from build123d import *

# Parameters (mm, degrees)
BOSS_EXTRUDE1_DEPTH = 19.05
SKETCH3_R           = 24.5745
CUT_EXTRUDE1_DEPTH  = 175.004260005
SKETCH5_R           = 51.3715
SKETCH5_R_2         = 46.5455
CUT_EXTRUDE2_DEPTH  = 2.794
SKETCH19_R          = 1.7272
CUT_EXTRUDE4_DEPTH  = 175.004260005
CIRPATTERN2_COUNT   = 8
SKETCH37_R          = 119.0625
SKETCH37_R_2        = 115.2525
CUT_EXTRUDE7_DEPTH  = 2.667
CIRPATTERN4_COUNT   = 8


with BuildPart() as part:
    # Sketch1 → Boss-Extrude1 (new body)
    with BuildSketch(Plane(origin=(0, 0, 0), x_dir=(1, 0, 0), z_dir=(0, 1, 0))):
        with BuildLine():
            ThreePointArc((-31.932272077, 122.3), (-48.371185851, 116.778372909), (-63.899633215, 109.058685463))
            Line((-63.899633215, 109.058685463), (-109.058685463, 63.899633215))
            ThreePointArc((-109.058685463, 63.899633215), (-116.778372909, 48.371185851), (-122.3, 31.932272077))
            Line((-122.3, 31.932272077), (-122.3, -31.932272077))
            ThreePointArc((-122.3, -31.932272077), (-116.778372909, -48.371185851), (-109.058685463, -63.899633215))
            Line((-109.058685463, -63.899633215), (-63.899633215, -109.058685463))
            ThreePointArc((-63.899633215, -109.058685463), (-48.371185851, -116.778372909), (-31.932272077, -122.3))
            Line((-31.932272077, -122.3), (31.932272077, -122.3))
            ThreePointArc((31.932272077, -122.3), (48.371185851, -116.778372909), (63.899633215, -109.058685463))
            Line((63.899633215, -109.058685463), (109.058685463, -63.899633215))
            ThreePointArc((109.058685463, -63.899633215), (116.778372909, -48.371185851), (122.3, -31.932272077))
            Line((122.3, -31.932272077), (122.3, 31.932272077))
            ThreePointArc((122.3, 31.932272077), (116.778372909, 48.371185851), (109.058685463, 63.899633215))
            Line((109.058685463, 63.899633215), (63.899633215, 109.058685463))
            ThreePointArc((63.899633215, 109.058685463), (48.371185851, 116.778372909), (31.932272077, 122.3))
            Line((31.932272077, 122.3), (-31.932272077, 122.3))
        make_face()
    extrude(amount=BOSS_EXTRUDE1_DEPTH)

    # Sketch3 → Cut-Extrude1 (cut, through all)
    with BuildSketch(Plane(origin=(0, 19.05, 0), x_dir=(1, 0, 0), z_dir=(0, 1, 0))):
        with Locations(Location((0, 0, 0), (0, 0, 270))):
            Circle(SKETCH3_R)
    extrude(amount=-CUT_EXTRUDE1_DEPTH, mode=Mode.SUBTRACT)

    # Sketch5 → Cut-Extrude2 (cut)
    with BuildSketch(Plane(origin=(0, 19.05, 0), x_dir=(1, 0, 0), z_dir=(0, 1, 0))):
        with Locations(Location((0, 0, 0), (0, 0, 270))):
            Circle(SKETCH5_R)
        with Locations(Location((0, 0, 0), (0, 0, 270))):
            Circle(SKETCH5_R_2, mode=Mode.SUBTRACT)
    extrude(amount=-CUT_EXTRUDE2_DEPTH, mode=Mode.SUBTRACT)

    # Sketch19 → Cut-Extrude4 (cut, through all)
    with BuildSketch(Plane(origin=(0, 19.05, 0), x_dir=(1, 0, 0), z_dir=(0, 1, 0))):
        with Locations(Location((-47.055461432, 113.601933173, 0), (0, 0, 270))):
            Circle(SKETCH19_R)
    cut_extrude4 = extrude(amount=-CUT_EXTRUDE4_DEPTH, mode=Mode.SUBTRACT)

    # CirPattern2: Cut-Extrude4 ×8 about axis
    cirpattern2_axis = Axis((0, 0, 0), (0, 1, 0))
    for i in range(1, CIRPATTERN2_COUNT):
        add(cut_extrude4.rotate(cirpattern2_axis, i * 360 / CIRPATTERN2_COUNT), mode=Mode.SUBTRACT)

    # Sketch23 → 5/16-18 Tapped Hole2 (revolve, cut)
    with BuildSketch(Plane(origin=(-71.374, 19.05, 0), x_dir=(0, 0, 1), z_dir=(1, 0, 0))):
        Polygon((0, 0), (0, 14.661148974), (3.2639, 12.7), (3.2639, 0), align=None)
    f_5_16_18_tapped_hole2 = revolve(axis=Axis((-71.374, 25.4, 0), (0, -1, 0)), mode=Mode.SUBTRACT)

    # Sketch37 → Cut-Extrude7 (cut)
    with BuildSketch(Plane.XZ):
        with Locations(Location((0, 0, 0), (0, 0, 270))):
            Circle(SKETCH37_R)
        with Locations(Location((0, 0, 0), (0, 0, 270))):
            Circle(SKETCH37_R_2, mode=Mode.SUBTRACT)
    extrude(amount=-CUT_EXTRUDE7_DEPTH, mode=Mode.SUBTRACT)

    # CirPattern4: 5/16-18 Tapped Hole2 ×8 about axis
    cirpattern4_axis = Axis((0, 0, 0), (0, 1, 0))
    for i in range(1, CIRPATTERN4_COUNT):
        add(f_5_16_18_tapped_hole2.rotate(cirpattern4_axis, i * 360 / CIRPATTERN4_COUNT), mode=Mode.SUBTRACT)


solid = part.part
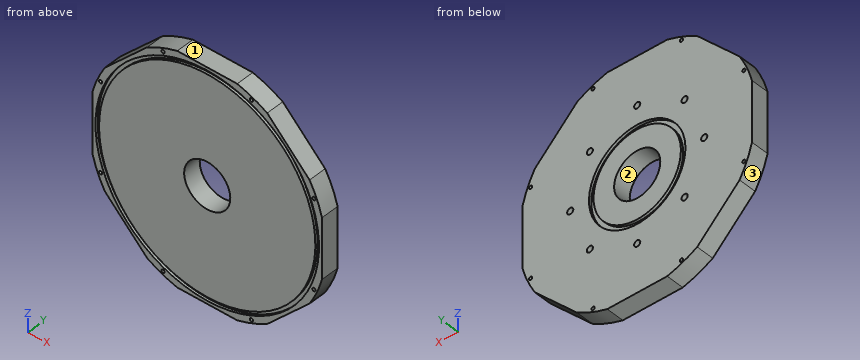
Geometry: final body of the model. Coordinates: model frame, mm. Face numbers are marked on the shaded views. Give positions to 0.01 mm unless a question says otherwise; leave off trailing zeros. Loops run counter-clockwise (first coordinate to the right, second up) from the corner with the lowest first, then second, coordinate; pieces in that order, holes last. Notation, with made-up numbers: (52.25, 77) -> (70.25, 77) arc R12 ccw to (70.25, 94) -> close; hole circle Ø11 at (-10, 66.25). An arc over 180 degrees is marked (long way). Put each result on its own line as item: value.
1. Ray query, line 1 along X through (y, z) = (18, 0); line 2 along X through (y, z) = (16.5, -13.5); line 3 along Z through (x, y) = (-50, 1.5). Return the intervals inside material, ascending. Write a range as [from, to].
Taken from the geometry:
line 1: x = [-122.3, -74.64], [-68.11, -51.37], [-46.55, -24.57], [24.57, 46.55], [51.37, 68.11], [74.64, 122.3]
line 2: x = [-122.3, -49.57], [-44.54, -20.53], [20.53, 44.54], [49.57, 122.3]
line 3: z = [-116.09, -108.05], [-103.84, 103.84], [108.05, 116.09]
2. Cut plane B-B (y = 10.5). Count the separate pieces of the cut face and the enclosed holes in it, plus the area to 3 significant figures.
Taken from the geometry:
separate pieces: 1
enclosed holes: 17
area: 46,600 mm2
3. Cut plane C-C (x = -13). Return the cut outline in (y, z), plus the area to 3 significant figures.
Taken from the geometry:
outline: (0, -122.3) -> (19.05, -122.3) -> (19.05, -49.7) -> (16.26, -49.7) -> (16.26, -44.69) -> (19.05, -44.69) -> (19.05, -20.85) -> (0, -20.85) -> (0, -114.52) -> (2.67, -114.52) -> (2.67, -118.35) -> (0, -118.35) -> close; (0, 20.85) -> (19.05, 20.85) -> (19.05, 44.69) -> (16.26, 44.69) -> (16.26, 49.7) -> (19.05, 49.7) -> (19.05, 122.3) -> (0, 122.3) -> (0, 118.35) -> (2.67, 118.35) -> (2.67, 114.52) -> (0, 114.52) -> close
area: 3,820 mm2
4. Cut plane A-A (z = 7.5). Return the cut outline in (x, y).
Taken from the geometry:
outline: (-122.3, 0) -> (-118.83, 0) -> (-118.83, 2.67) -> (-115.01, 2.67) -> (-115.01, 0) -> (-23.4, 0) -> (-23.4, 19.05) -> (-45.94, 19.05) -> (-45.94, 16.26) -> (-50.82, 16.26) -> (-50.82, 19.05) -> (-122.3, 19.05) -> close; (23.4, 0) -> (115.01, 0) -> (115.01, 2.67) -> (118.83, 2.67) -> (118.83, 0) -> (122.3, 0) -> (122.3, 19.05) -> (50.82, 19.05) -> (50.82, 16.26) -> (45.94, 16.26) -> (45.94, 19.05) -> (23.4, 19.05) -> close
5. Cut plane D-D (x = 61). Return the cut outline in (y, z).
Taken from the geometry:
outline: (0, -110.71) -> (19.05, -110.71) -> (19.05, 110.71) -> (0, 110.71) -> (0, 102.25) -> (2.67, 102.25) -> (2.67, 97.79) -> (0, 97.79) -> (0, -97.79) -> (2.67, -97.79) -> (2.67, -102.25) -> (0, -102.25) -> close
6. Pin query (flat end, axial travel): P1, Ø1.5, axis at x = -38.5, y = 12, coming from the +Z side; P2, Ø4, axis at y = 2, z = 63.5, coming from the +X side; P3, Ø8, axis at x = -92, y = 7, coming from the +Z side; P4, Ø1, axis at x = -77.5, z = -96.5, coming from the +Y side. Return the tip coordinate at first contact, or that it passes through.
Taken from the geometry:
P1: stops at z = 120.63
P2: stops at x = 110.43
P3: stops at z = 84.96
P4: passes through
7. Pull-direction query (Z, two-part tool) for the marked faces 1, 2 and 3; classes: released by +Z, released by -Z, zero draft, split by the parting line, or undercut.
Taken from the geometry:
face 1: released by +Z
face 2: undercut
face 3: released by -Z
